from build123d import *

# Parameters (mm, degrees)
SKETCH_R        = 4.5
PAD_DEPTH       = 2
SKETCH001_R     = 5.5
PAD001_DEPTH    = 2
SKETCH003_W     = 13
SKETCH003_H     = 13
PAD002_DEPTH    = 16
POCKET_DEPTH    = 20
SKETCH005_W     = 4.5
SKETCH005_H     = 2.303615
POCKET001_DEPTH = 7


with BuildPart() as part:
    # Sketch → Pad (new body)
    with BuildSketch(Plane.XY):
        Circle(SKETCH_R)
    extrude(amount=PAD_DEPTH)

    # Sketch001 (on Face3 of Pad) → Pad001 (join)
    with BuildSketch(Plane.XY.offset(2)):
        Circle(SKETCH001_R)
    extrude(amount=PAD001_DEPTH)

    # Sketch003 (on Face3 of Pad001) → Pad002 (join)
    with BuildSketch(Plane.XY.offset(4)):
        Rectangle(SKETCH003_W, SKETCH003_H)
    extrude(amount=PAD002_DEPTH)

    # Sketch004 (on Face10 of Pad002) → Pocket (cut)
    with BuildSketch(Plane(origin=(0, 0, 0), x_dir=(1, 0, 0), z_dir=(0, 0, -1))):
        with BuildLine():
            ThreePointArc((-3.2, 1.75), (-4.95, 0), (-3.2, -1.75))
            Line((-3.2, -1.75), (3.2, -1.75))
            ThreePointArc((3.2, -1.75), (4.95, 0), (3.2, 1.75))
            Line((-3.2, 1.75), (3.2, 1.75))
        make_face()
    extrude(amount=-POCKET_DEPTH, mode=Mode.SUBTRACT)

    # Sketch005 (on Face5 of Pocket) → Pocket001 (cut)
    with BuildSketch(Plane.XY.offset(20)):
        with Locations((0, 1.879977)):
            Rectangle(SKETCH005_W, SKETCH005_H)
    extrude(amount=-POCKET001_DEPTH, mode=Mode.SUBTRACT)


solid = part.part
Verification items for the finished model (mm, model axes). A direction names the side the tool comes from. Round coordinates to 2 decimals unless told otherwise and drop trailing zeros. Write each loop counter-clockwise with the first axis right and the second up, starting at its lowest first coordinate (ties: lowest second). Pieces come first, ordered by that corner, then holes.
(1) Section check D-D (x = -2). Enter the section's corners in (y, z), plus the area to 3 significant figures.
Returned:
outline: (-6.5, 4) - (-5.12, 4) - (-5.12, 2) - (-4.03, 2) - (-4.03, 0) - (-1.75, 0) - (-1.75, 20) - (-6.5, 20) - close; (1.75, 0) - (4.03, 0) - (4.03, 2) - (5.12, 2) - (5.12, 4) - (6.5, 4) - (6.5, 20) - (3.03, 20) - (3.03, 13) - (1.75, 13) - close
area: 166 mm2
(2) Mould release check, pull along X, two halves, no side actions. Record for faces 5 (the flat face through (0, 3.032, 17)), 6 (the flat face through (-1.2, -4.5, 2)), 7 (the flat face through (-6.5, 0, 12)), 8 (the cylindrical face through (-4.95, -0.04, 9.86)): pulls with the +X half, pulls with the -X half, needs draft (parallel to the pull), parting line crosses it, or undercut.
Returned:
face 5: undercut
face 6: needs draft
face 7: pulls with the -X half
face 8: undercut
(3) Section check A-A (x = 0). Enter the section's corners in (y, z), plus the area to 3 significant figures.
Returned:
outline: (-6.5, 4) - (-5.5, 4) - (-5.5, 2) - (-4.5, 2) - (-4.5, 0) - (-1.75, 0) - (-1.75, 20) - (-6.5, 20) - close; (1.75, 0) - (4.5, 0) - (4.5, 2) - (5.5, 2) - (5.5, 4) - (6.5, 4) - (6.5, 20) - (3.03, 20) - (3.03, 13) - (1.75, 13) - close
area: 169 mm2
(4) Depth check by flat-ended pin: pin 1 Ø3.5 at (x, y) = (1.5, 1.5) entering from -Z. Enter the tip coordinate at first touch or a pass-through.
Returned:
pin 1: stops at z = 0
(5) Access from +Z, -Z, +X, -X, +Y, -Y to the whole of each face (thin tool, end or side, straight path). Record for faces 1 (the cylindrical face through (-1.19, -5.37, 2.99)), 2 (the flat face through (2.25, 2, 17)), 3 (the cylindrical face through (-0.1, -4.5, 1)), 4 (the cylindrical face through (0.1, 4.5, 1)).
Returned:
face 1: -Z
face 2: +Z
face 3: -Z, -Y
face 4: -Z, +Y
(6) Section check B-B (y = 0). Enter the section's corners in (x, z).
Returned:
outline: (-6.5, 4) - (-5.5, 4) - (-5.5, 2) - (-4.95, 2) - (-4.95, 20) - (-6.5, 20) - close; (4.95, 2) - (5.5, 2) - (5.5, 4) - (6.5, 4) - (6.5, 20) - (4.95, 20) - close
(7) Section check C-C (z = 13.75). Enter the section's corners in (x, y).
Returned:
outline: (-6.5, -6.5) - (6.5, -6.5) - (6.5, 6.5) - (-6.5, 6.5) - close; hole (-3.2, -1.75) - (3.2, -1.75) arc R1.75 ccw to (3.2, 1.75) - (2.25, 1.75) - (2.25, 3.03) - (-2.25, 3.03) - (-2.25, 1.75) - (-3.2, 1.75) arc R1.75 ccw to start
(8) Material ranges on line 1 (Y direction, x = 1.5, z = 16); line 2 (Y direction, x = -1.25, z = 11.5); line 3 (X direction, y = -1.5, z = 12.25), recorded low to high.
Returned:
line 1: y = -6.5 to -1.75, 3.03 to 6.5
line 2: y = -6.5 to -1.75, 1.75 to 6.5
line 3: x = -6.5 to -4.1, 4.1 to 6.5
